Part print with two shaded views. Sizes in mm from the minimum x, y, z corner. Round coordinates to 2 decimals unless told otherwise and drop trailing zeros. Order: outer loops, then holes, each group sorted by start corner. A loop starts at its lowest first (then second) coordinate and runs counter-clockwise, first axis right, second up. Notation, with made-up numbers: M -1.5,-7 L 51.5,-7 A15 ccw 51.5,6 Z; hole C 40,67.5 d1. An arc over 180 degrees is marked long. Answer as a JSON object with one key per item and string values.
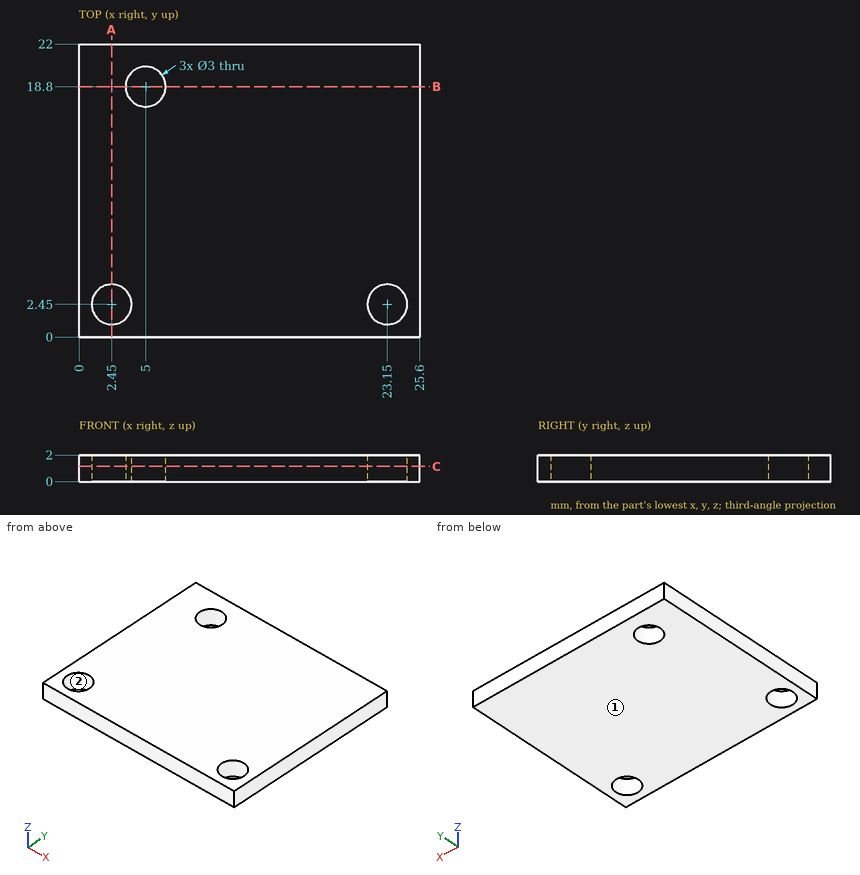
Item 1: Saw through at A-A on x = 2.45. List the corners of the cut face in (y, z).
Worked answers:
{"outline": "M 0,0 L 0.95,0 L 0.95,2 L 0,2 Z; M 3.95,0 L 22,0 L 22,2 L 3.95,2 Z"}
Item 2: Two-plate mould, pull along Y, no slides. Class the marked faces 1 and 2: released by +Y, released by -Y, zero draft, split by the parting line, or undercut.
Worked answers:
{"face 1": "zero draft", "face 2": "undercut"}
Item 3: Wall check: line 1 along Y through (x, z) = (5, 1.7); line 2 along Y through (x, z) = (2.45, 0.4); line 3 along X through (y, z) = (19.5, 0.4). Give the ranges that are in metal, low to high. Write a range as [from, to].
Worked answers:
{"line 1": "y = [0, 17.3], [20.3, 22]", "line 2": "y = [0, 0.95], [3.95, 22]", "line 3": "x = [0, 3.67], [6.33, 25.6]"}
Item 4: Saw through at B-B on y = 18.8. List the corners of the cut face in (x, z).
Worked answers:
{"outline": "M 0,0 L 3.5,0 L 3.5,2 L 0,2 Z; M 6.5,0 L 25.6,0 L 25.6,2 L 6.5,2 Z"}
Item 5: Saw through at C-C on z = 1.15. List the corners of the cut face in (x, y).
Worked answers:
{"outline": "M 0,0 L 25.6,0 L 25.6,22 L 0,22 Z; hole C 2.45,2.45 d3; hole C 5,18.8 d3; hole C 23.15,2.45 d3"}
Item 6: Drop a flat-ended pin along its axis: pin 1 Ø1.8 at (x, y) = (5, 18.8) entering from +Z. Give the stop position or say it passes through.
Worked answers:
{"pin 1": "passes through"}
